The model under review builds one solid part; all positions refer to its coordinate system, in mm. A direction names the side the tool comes from. Give positions to 0.01 mm unless a question says otherwise; leave off trailing zeros. Order: outer loops, then holes, each group sorted by start corner. A loop starts at its lowest first (then second) coordinate and runs counter-clockwise, first axis right, second up. Notation, with made-up numbers: (73.25, -15) - (127.25, -15) arc R25 cw to (127.25, 16) - close; hole circle Ø6 at (-34.75, 8). An arc over 180 degrees is marked (long way). Put each result on its own line as item: value.
```python
from build123d import *

# Parameters (mm, degrees)
F0_W          = 203.2
F0_H          = 101.6
F1_DEPTH      = 25.4
F1_DEPTH_BACK = 25.4
F2_T          = -5.08
F3_R          = 7.363312
F3_R_2        = 6.379647
F4_DEPTH      = 101.601


with BuildPart() as f1:
    # F0 (on Top) → F1 (new body, two sides)
    with BuildSketch(Plane.XY) as f1_sk:
        Rectangle(F0_W, F0_H)
    extrude(amount=F1_DEPTH)
    extrude(f1_sk.sketch, amount=-F1_DEPTH_BACK)

    # F2
    f2_openings = [f1.faces().sort_by_distance(p)[0] for p in [
        (0, 0, 25.4),
    ]]
    offset(amount=F2_T, openings=f2_openings)

    # F3 (on face) → F4 (cut, through all)
    with BuildSketch(Plane.XZ.offset(50.8)):
        with Locations((-61.689176, 8.265927)):
            Circle(F3_R)
        with Locations((43.166649, -7.2081)):
            Circle(F3_R_2)
    extrude(amount=-F4_DEPTH, mode=Mode.SUBTRACT)


solid = f1.part
```
(1) Take a section at B-B, the plane x = 12.5. Write out the cut boundary in (y, z), then the cut area to 3 significant figures.
The answers:
outline: (-50.8, -25.4) - (50.8, -25.4) - (50.8, 25.4) - (45.72, 25.4) - (45.72, -20.32) - (-45.72, -20.32) - (-45.72, 25.4) - (-50.8, 25.4) - close
area: 981 mm^2
(2) Take a section at A-A, the plane z = -16. Write out the cut boundary in (x, y).
The answers:
outline: (-101.6, -50.8) - (101.6, -50.8) - (101.6, 50.8) - (-101.6, 50.8) - close; hole (-96.52, -45.72) - (96.52, -45.72) - (96.52, 45.72) - (-96.52, 45.72) - close
(3) Clearance check with a flat-ended pin moving along its axis: pin 1 Ø1 at (x, y) = (-63.5, -35) entering from +Z. State where the tip first meets the part, or that it passes through.
The answers:
pin 1: z = -20.32
(4) Take a section at C-C, the plane y = 40.5. Write out the cut boundary in (x, z).
The answers:
outline: (-101.6, -25.4) - (101.6, -25.4) - (101.6, 25.4) - (96.52, 25.4) - (96.52, -20.32) - (-96.52, -20.32) - (-96.52, 25.4) - (-101.6, 25.4) - close
(5) Take a section at D-D, the plane z = 4.5. Write out the cut boundary in (x, y).
The answers:
outline: (-101.6, -50.8) - (-68.02, -50.8) - (-68.02, -45.72) - (-96.52, -45.72) - (-96.52, 45.72) - (-68.02, 45.72) - (-68.02, 50.8) - (-101.6, 50.8) - close; (-55.36, -50.8) - (101.6, -50.8) - (101.6, 50.8) - (-55.36, 50.8) - (-55.36, 45.72) - (96.52, 45.72) - (96.52, -45.72) - (-55.36, -45.72) - close
(6) Wall thickness on L1, parallel to X at y = -9.5, z = 15; L2, parallel to Y at x = -45.5, z = 8; L3, parallel to Z at x = 45, y = 39: over which ranges is each line inside the solid? List them lowest first.
The answers:
L1: -101.6 to -96.52, 96.52 to 101.6
L2: -50.8 to -45.72, 45.72 to 50.8
L3: -25.4 to -20.32
(7) For faces 1 (the flat face through (-8, -49, 25.4)), 2 (the flat face through (96.52, -1, 3)), list the 3-axis set-ups (+Z, -Z, +X, -X, +Y, -Y) from which the entire face can be reached by the end or side of a thin tool; tool diameter is ignored.
The answers:
face 1: +Z, +X, -X, +Y, -Y
face 2: +Z
(8) The part is to be moulded in two halves that separate along Y. For faces 3 (the flat face through (-1, 45.72, 3)), 4 (the flat face through (-101.6, -1, 0)), 5 (the flat face through (-1, -50.8, 0)), say which applies: pulls with the +Y half, pulls with the -Y half, needs draft (parallel to the pull), parting line crosses it, or undercut.
The answers:
face 3: undercut
face 4: needs draft
face 5: pulls with the -Y half
